Source: CAD feature listing. Evaluate the final solid. Frame: model axes, mm. A direction names the side the tool comes from. Coordinates: 2 decimals unless noted, no trailing zeros. Order: outer loops, then holes, each group sorted by start corner. A loop starts at its lowest first (then second) coordinate and runs counter-clockwise, first axis right, second up. Notation, with made-up numbers: (75, 70.5) - (91, 70.5) arc R23 cw to (91, 83.5) - close; hole circle Ø2 at (-11.5, -8). An arc over 180 degrees is marked (long way). One line per question, with ' | ' between items.
from build123d import *

# Parameters (mm, degrees)
SKETCH1_R           = 2.5
BOSS_EXTRUDE1_DEPTH = 10
SKETCH2_R           = 4
BOSS_EXTRUDE2_DEPTH = 4
CUT_EXTRUDE1_DEPTH  = 3


with BuildPart() as part:
    # Sketch1 → Boss-Extrude1 (new body)
    with BuildSketch(Plane.XY):
        Circle(SKETCH1_R)
    extrude(amount=BOSS_EXTRUDE1_DEPTH)

    # Sketch2 → Boss-Extrude2 (add)
    with BuildSketch(Plane(origin=(0, 0, 0), x_dir=(-1, 0, 0), z_dir=(0, 0, -1))):
        Circle(SKETCH2_R)
    extrude(amount=BOSS_EXTRUDE2_DEPTH)

    # Sketch3 → Cut-Extrude1 (cut)
    with BuildSketch(Plane(origin=(0, 0, -4), x_dir=(-1, 0, 0), z_dir=(0, 0, -1))):
        Polygon((1.732050808, -3), (3.464101615, 0), (1.732050808, 3), (-1.732050808, 3), (-3.464101615, 0), (-1.732050808, -3), align=None)
    extrude(amount=-CUT_EXTRUDE1_DEPTH, mode=Mode.SUBTRACT)


solid = part.part
(1) Cut plane D-D (x = 3). Return the cut outline in (y, z).
Taken from the geometry:
outline: (-2.65, -4) - (-0.8, -4) - (-0.8, -1) - (0.8, -1) - (0.8, -4) - (2.65, -4) - (2.65, 0) - (-2.65, 0) - close
(2) Pin query (flat end, axial travel): P1, Ø3, axis at x = 0, y = 0, coming from the -Z side; P2, Ø4, axis at x = 0, z = 6.5, coming from the +Y side. Return the tip coordinate at first contact, or that it passes through.
Taken from the geometry:
P1: stops at z = -1 | P2: stops at y = 2.5
(3) Pull-direction query (Y, two-part tool) for faces 1 (the flat face through (-2.6, 1.5, -2.5)), 2 (the flat face through (0, 0, 10)), 3 (the cylindrical face through (-0.54, -2.44, 4.93)); classes: pulls with the +Y half, pulls with the -Y half, needs draft (parallel to the pull), parting line crosses it, or undercut.
Taken from the geometry:
face 1: undercut | face 2: needs draft | face 3: parting line crosses it
(4) Material intervals for L1, parallel to Z at x = 2.75, y = 1; L2, parallel to Z at x = 1.5, y = -1.75; L3, parallel to Y at x = 0, z = 8.5, sorted ascending. Write a range as from..to.
Taken from the geometry:
L1: z = -1..0 | L2: z = -1..10 | L3: y = -2.5..2.5
(5) Cut plane C-C (z = 1.5). Return the cut outline in (x, y), and give its area (3 significant figures).
Taken from the geometry:
outline: circle Ø5 at (0, 0) | area: 19.6 mm²
(6) Cut plane B-B (y = 1.5). Return the cut outline in (x, z), and give its area (3 significant figures).
Taken from the geometry:
outline: (-3.71, -4) - (-2.6, -4) - (-2.6, -1) - (2.6, -1) - (2.6, -4) - (3.71, -4) - (3.71, 0) - (2, 0) - (2, 10) - (-2, 10) - (-2, 0) - (-3.71, 0) - close | area: 54.1 mm²
(7) Set-up query: faces 4 (the flat face through (-2, 2, 0)), 5 (the flat face through (2.6, -1.5, -2.5)), 6 (the flat face through (-3, 2, -4)). Return all of +Z, -Z, +X, -X, +Y, -Y with unobstructed straight access to the full face (end or side cutting, diameter ignored); none if empty.
Taken from the geometry:
face 4: +Z | face 5: -Z | face 6: -Z, +X, -X, +Y, -Y
(8) Cut plane A-A (x = 0). Return the cut outline in (y, z), and give its area (3 significant figures).
Taken from the geometry:
outline: (-4, -4) - (-3, -4) - (-3, -1) - (3, -1) - (3, -4) - (4, -4) - (4, 0) - (2.5, 0) - (2.5, 10) - (-2.5, 10) - (-2.5, 0) - (-4, 0) - close | area: 64.0 mm²
